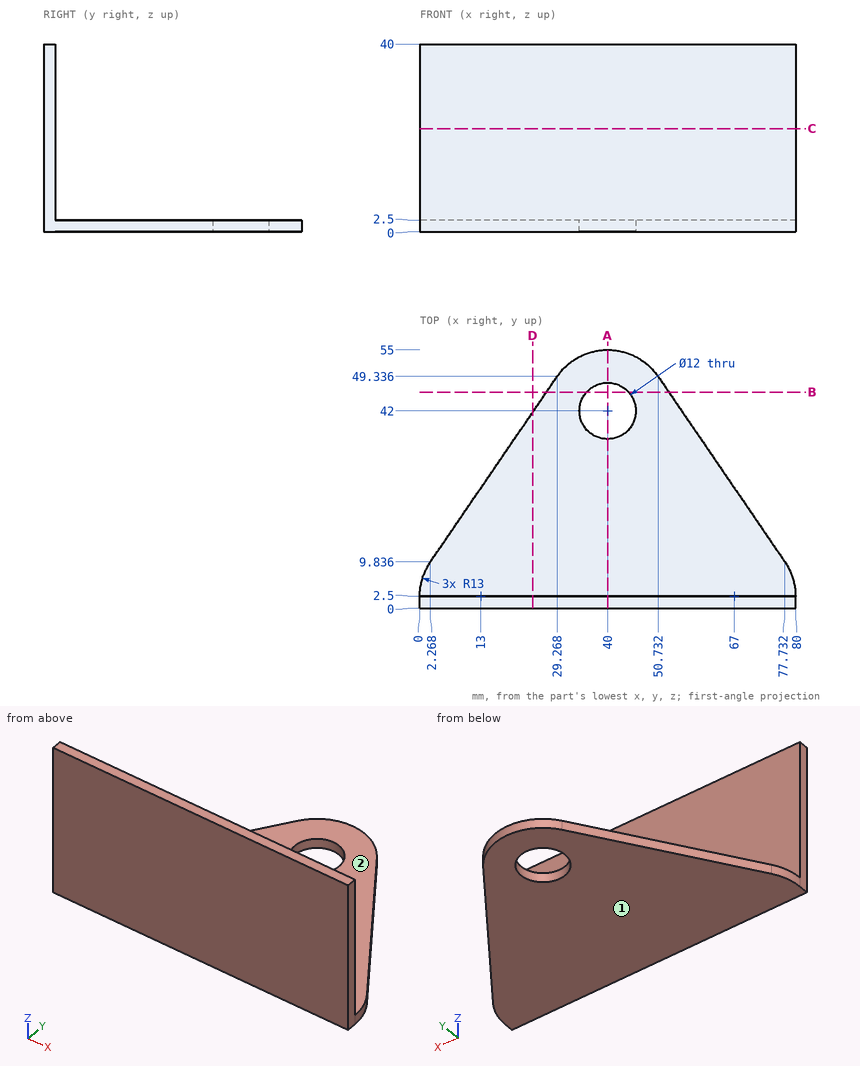
Source: three-view drawing plus pictorial views. Frame: mm from the lowest corner of the part. A direction names the side the tool comes from. Round coordinates to 2 decimals unless told otherwise and drop trailing zeros. Loops run counter-clockwise (first coordinate to the right, second up) from the corner with the lowest first, then second, coordinate; pieces in that order, holes last.
Q1. Section D-D on x = 24. Return loops of the section in (y, z).
Q2. Pin query (flat end, axial travel): P1, Ø6, axis at x = 22.5, z = 35.5, coming from the +Y side; P2, Ø8, axis at x = 17, y = 18, coming from the +Z side; P3, Ø9.5, axis at x = 40, y = 42, coming from the -Z side. Return the tip coordinate at first contact, or that it passes through.
Q3. Section B-B on y = 46. Return loops of the section in (x, z).
Q4. Section A-A on x = 40. Return loops of the section in (y, z).
Q5. Material intervals for L1, parallel to Y at x = 40, z = 1; L2, parallel to Y at x = 53, z = 37, sorted ascending.
Q6. Access query for the marked faces 1 and 2. Directions: +Z, -Z, +X, -X, +Y, -Y. A direction counts if a zero-diameter tool reaches every point of the face in a straight line with its end or side. Return the directions, or none.
Q7. Section C-C on z = 22. Return loops of the section in (x, y).
Evaluation:
1. outline: (0, 0) - (41.63, 0) - (41.63, 2.5) - (2.5, 2.5) - (2.5, 40) - (0, 40) - close
2. P1: stops at y = 2.5
2. P2: stops at z = 2.5
2. P3: passes through
3. outline: (26.99, 0) - (35.53, 0) - (35.53, 2.5) - (26.99, 2.5) - close; (44.47, 0) - (53.01, 0) - (53.01, 2.5) - (44.47, 2.5) - close
4. outline: (0, 0) - (36, 0) - (36, 2.5) - (2.5, 2.5) - (2.5, 40) - (0, 40) - close; (48, 0) - (55, 0) - (55, 2.5) - (48, 2.5) - close
5. L1: y = 0 to 36, 48 to 55
5. L2: y = 0 to 2.5
6. face 1: -Z, +X, -X, +Y, -Y
6. face 2: +Z, +X, -X, +Y
7. outline: (0, 0) - (80, 0) - (80, 2.5) - (0, 2.5) - close
